```python
from build123d import *

# Parameters (mm, degrees)
SKETCH1_R            = 4
BOSS_EXTRUDE1_DEPTH  = 2.5
CUT_EXTRUDE1_DEPTH   = 10
FILLET1_R            = 2.5
FILLET2_R            = 1
M3_CLEARANCE_HOLE1_D = 3.4
M3_CLEARANCE_HOLE2_D = 3.4


with BuildPart() as part:
    # Sketch1 → Boss-Extrude1 (new, symmetric)
    with BuildSketch(Plane(origin=(0, 0, 0), x_dir=(1, 0, 0), z_dir=(0, 1, 0))):
        with BuildLine():
            Line((0, 37.5), (0, 45))
            Line((0, 45), (21.25988463, 45))
            ThreePointArc((21.25988463, 45), (32.740387601, 47.283614025), (42.473088065, 53.786796564))
            Line((42.473088065, 53.786796564), (60.630111199, 71.943819698))
            ThreePointArc((60.630111199, 71.943819698), (62.864579349, 75.353330401), (63.552689718, 79.371304426))
            ThreePointArc((63.552689718, 79.371304426), (65.137560566, 83.204452196), (69.070514812, 84.522294498))
            ThreePointArc((69.070514812, 84.522294498), (70.16592161, 84.652219255), (71.098782729, 85.240918353))
            Line((71.098782729, 85.240918353), (73.858107414, 88.000243038))
            ThreePointArc((73.858107414, 88.000243038), (74.446806512, 88.933104157), (74.576731268, 90.028510955))
            ThreePointArc((74.576731268, 90.028510955), (76.231825981, 94.29022854), (80.660715996, 95.424472129))
            ThreePointArc((80.660715996, 95.424472129), (86.294292266, 94.799388668), (91.923881554, 95.45941546))
            Line((91.923881554, 95.45941546), (95.45941546, 91.923881554))
            ThreePointArc((95.45941546, 91.923881554), (94.799388668, 86.294292266), (95.424472129, 80.660715996))
            ThreePointArc((95.424472129, 80.660715996), (94.29022854, 76.231825981), (90.028510955, 74.576731268))
            ThreePointArc((90.028510955, 74.576731268), (88.933104157, 74.446806512), (88.000243038, 73.858107414))
            Line((88.000243038, 73.858107414), (85.240918353, 71.098782729))
            ThreePointArc((85.240918353, 71.098782729), (84.652219255, 70.16592161), (84.522294498, 69.070514812))
            ThreePointArc((84.522294498, 69.070514812), (83.204452196, 65.137560566), (79.371304426, 63.552689718))
            ThreePointArc((79.371304426, 63.552689718), (75.353330401, 62.864579349), (71.943819698, 60.630111199))
            Line((71.943819698, 60.630111199), (41.715728753, 30.402020254))
            ThreePointArc((41.715728753, 30.402020254), (33.0448187, 17.425086301), (30, 2.117749006))
            Line((30, 2.117749006), (30, 0))
            Line((30, 0), (22.5, 0))
            Line((22.5, 0), (22.5, 5))
            Line((22.5, 5), (15, 5))
            Line((15, 5), (15, 30))
            Line((15, 30), (5, 30))
            Line((5, 30), (5, 37.5))
            Line((5, 37.5), (0, 37.5))
        make_face()
        with Locations(Location((79.549512883, 79.549512883, 0), (0, 0, 270))):
            Circle(SKETCH1_R, mode=Mode.SUBTRACT)
        with BuildLine():
            Line((77.849512883, 87.549512883), (77.849512883, 90.549512883))
            ThreePointArc((77.849512883, 90.549512883), (79.549512883, 92.249512883), (81.249512883, 90.549512883))
            Line((81.249512883, 90.549512883), (81.249512883, 87.549512883))
            ThreePointArc((81.249512883, 87.549512883), (79.549512883, 85.849512883), (77.849512883, 87.549512883))
        make_face(mode=Mode.SUBTRACT)
        with BuildLine():
            Line((87.549512883, 81.249512883), (90.549512883, 81.249512883))
            ThreePointArc((90.549512883, 81.249512883), (92.249512883, 79.549512883), (90.549512883, 77.849512883))
            Line((90.549512883, 77.849512883), (87.549512883, 77.849512883))
            ThreePointArc((87.549512883, 77.849512883), (85.849512883, 79.549512883), (87.549512883, 81.249512883))
        make_face(mode=Mode.SUBTRACT)
        with BuildLine():
            Line((81.249512883, 71.549512883), (81.249512883, 68.549512883))
            ThreePointArc((81.249512883, 68.549512883), (79.549512883, 66.849512883), (77.849512883, 68.549512883))
            Line((77.849512883, 68.549512883), (77.849512883, 71.549512883))
            ThreePointArc((77.849512883, 71.549512883), (79.549512883, 73.249512883), (81.249512883, 71.549512883))
        make_face(mode=Mode.SUBTRACT)
        with BuildLine():
            Line((71.549512883, 77.849512883), (68.549512883, 77.849512883))
            ThreePointArc((68.549512883, 77.849512883), (66.849512883, 79.549512883), (68.549512883, 81.249512883))
            Line((68.549512883, 81.249512883), (71.549512883, 81.249512883))
            ThreePointArc((71.549512883, 81.249512883), (73.249512883, 79.549512883), (71.549512883, 77.849512883))
        make_face(mode=Mode.SUBTRACT)
    extrude(amount=BOSS_EXTRUDE1_DEPTH, both=True)

    # Sketch2 → Cut-Extrude1 (cut)
    with BuildSketch(Plane(origin=(0, 2.5, 0), x_dir=(1, 0, 0), z_dir=(0, 1, 0))):
        Polygon((21, 24), (15, 30), (15, 8), (21, 14), align=None)
    extrude(amount=-CUT_EXTRUDE1_DEPTH, mode=Mode.SUBTRACT)

    # Fillet1
    fillet1_edges = [part.edges().sort_by_distance(p)[0] for p in [
        (91.923881554, 0, -95.45941546),
        (95.45941546, 0, -91.923881554),
    ]]
    fillet(fillet1_edges, radius=FILLET1_R)

    # Fillet2
    fillet2_edges = [part.edges().sort_by_distance(p)[0] for p in [
        (21, 0, -14),
        (15, 0, -8),
        (21, 0, -24),
        (30, 0, 0),
        (22.5, 0, 0),
        (22.5, 0, -5),
        (15, 0, -5),
        (15, 0, -30),
        (5, 0, -30),
        (5, 0, -37.5),
        (0, 0, -37.5),
        (0, 0, -45),
    ]]
    fillet(fillet2_edges, radius=FILLET2_R)

    # M3 Clearance Hole1 (through all)
    with Locations(Plane(origin=(0, 2.5, 0), x_dir=(1, 0, 0), z_dir=(0, 1, 0))):
        with Locations((35, 35)):
            Hole(M3_CLEARANCE_HOLE1_D / 2)

    # M3 Clearance Hole2 (through all)
    with Locations(Plane(origin=(0, 2.5, 0), x_dir=(1, 0, 0), z_dir=(0, 1, 0))):
        with Locations((12.5, 37.5), (25, 10)):
            Hole(M3_CLEARANCE_HOLE2_D / 2)


solid = part.part
```
Geometry check sheet. Reference: the model listing, model coordinates, mm. A direction names the side the tool comes from. Coordinates: 2 decimals unless noted, no trailing zeros. Order: outer loops, then holes, each group sorted by start corner. A loop starts at its lowest first (then second) coordinate and runs counter-clockwise, first axis right, second up. Notation, with made-up numbers: (3.5, -9) - (53.5, -9) arc R17 ccw to (53.5, -2) - close; hole circle Ø11 at (-12.5, 80). An arc over 180 degrees is marked (long way). Answer in a Markdown table with one row per item. Add a question column.
1. Section check B-B (z = -10). Enter the section's corners in (x, y), plus the area to 3 significant figures.
2. Material ranges on L1, parallel to X at y = 1.65, z = -78; L2, parallel to X at y = 0.95, z = -35; L3, parallel to Z at x = 11.5, y = -1.85, recorded low to high. Write a range as [from, to].
3. Section check A-A (x = 12.5). Enter the section's corners in (y, z), plus the area to 3 significant figures.
4. Gauge pin test, flat ends, axial feed: pin 1 Ø3 at (y, z) = (0.5, -80.5) entering from -X; pin 2 Ø0.6 at (y, z) = (-1, -1.5) entering from +X; pin 3 Ø1.5 at (x, y) = (70.5, -0.5) entering from -Z. Record the tip position at first contact, or that the pin passes through.
5. Section check D-D (x = 65.5). Enter the section's corners in (y, z), plus the area to 3 significant figures.
6. Draft check along Z on faces 4 (the face through (0, 0, -41)), 5 (the face through (85.85, 0.04, -79.51)), 6 (the face through (75.407, 0.035, -62.885)), 7 (the face through (32.59, 0.04, -47.22)). Enter one of: +Z half, -Z half, draft (parallel to the pull), parting line (faces both ways), or undercut.
7. Access from +Z, -Z, +X, -X, +Y, -Y to the whole of each face (thin tool, end or side, straight path). Record for faces 1 (the face through (79.51, 0.04, -73.25)), 2 (the face through (21, 0, -19)), 3 (the face through (11, 0, -45)).
8. Section check C-C (y = 1.25). Give the number of separate pieces and of enclosed holes in the cut face, plus the area to 3 significant figures.
Data:
| question | item | result |
|---|---|---|
| 1 | outline | (17, -2.5) - (23.3, -2.5) - (23.3, 2.5) - (17, 2.5) - close; (26.7, -2.5) - (30.78, -2.5) - (30.78, 2.5) - (26.7, 2.5) - close |
| 1 | area | 51.9 mm² |
| 2 | L1 | x = [63.51, 67.85], [72.25, 75.86], [83.24, 86.85], [91.25, 95.3] |
| 2 | L2 | x = [5, 33.3], [36.7, 46.31] |
| 2 | L3 | z = [-45, -38.87], [-36.13, -30] |
| 3 | outline | (-2.5, -45) - (2.5, -45) - (2.5, -39.2) - (-2.5, -39.2) - close; (-2.5, -35.8) - (2.5, -35.8) - (2.5, -30) - (-2.5, -30) - close |
| 3 | area | 58.0 mm² |
| 4 | pin 1 | stops at x = 63.55 |
| 4 | pin 2 | stops at x = 30 |
| 4 | pin 3 | stops at z = -85.39 |
| 5 | outline | (-2.5, -83.51) - (2.5, -83.51) - (2.5, -54.19) - (-2.5, -54.19) - close |
| 5 | area | 147 mm² |
| 6 | face 4 | draft |
| 6 | face 5 | undercut |
| 6 | face 6 | +Z half |
| 6 | face 7 | -Z half |
| 7 | face 1 | +Y, -Y |
| 7 | face 2 | -X, +Y, -Y |
| 7 | face 3 | -Z, -X, +Y, -Y |
| 8 | separate pieces | 1 |
| 8 | enclosed holes | 8 |
| 8 | area | 2,220 mm² |
